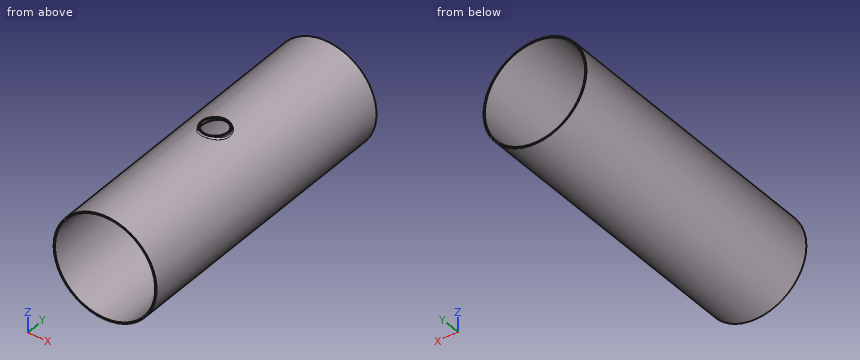
Autodesk Inventor part; units mm, degrees
ref_plane "YZ Plane" through (0, 0, 0) normal (1, 0, 0) x (0, 1, 0)
ref_plane "XZ Plane" through (0, 0, 0) normal (0, 1, 0) x (-1, 0, 0)
ref_plane "XY Plane" through (0, 0, 0) normal (0, 0, 1) x (1, 0, 0)
sketch "Szkic8" plane through (0, 0, 0) normal (0, 1, 0) x (-1, 0, 0)
  circle A0 centre (0, 0) radius 77
  circle A1 centre (0, 0) radius 75
  dimension "d53" = 154
  dimension "d54" = 2
extrude "Wyciągnięcie proste2" add sketch "Szkic8" along normal mid plane 450
sketch "Szkic13" plane through (0, 0, 0) normal (0, 0, 1) x (1, 0, 0)
  circle A0 centre (0, 0) radius 20.5
  circle A1 centre (0, 0) radius 18.5
  dimension "d67" = 41
  dimension "d68" = 2
extrude "Wyciągnięcie proste6" add sketch "Szkic13" along normal blind 79
sketch "Szkic14" plane through (0, 0, 79) normal (0, 0, 1) x (1, 0, 0)
  circle A0 centre (0, 0) radius 18.5
extrude "Wyciągnięcie proste7" cut sketch "Szkic14" against normal blind 79
sketch "Szkic15" plane through (0, -225, 0) normal (0, -1, 0) x (1, 0, 0)
  circle A0 centre (0, 0) radius 75
extrude "Wyciągnięcie proste8" cut sketch "Szkic15" against normal blind 450
fillet "Zaokrąglenie3" radius 2 2 edges at (0, 20.5, 77) (-0.0041, -20.5, 77)
fillet "Zaokrąglenie4" radius 4 2 edges at (-0.0039, -18.5, 75) (0, 18.5, 75)
equation "\"d53\" = OD"
equation "\"d54\" = THK"
equation "\"d55\" = L1"
equation "\"d67\" = OD2"
equation "\"d68\" = THK"
equation "\"d69\" = L2"
equation "\"d71\" = L2"
equation "\"d73\" = L1"
equation "\"d75\" = THK"
equation "\"d76\" = 2 * THK"
equation "\"SzerokośćGięciaPodcięcia\" = Grubość"
equation "\"RozmiarPodcięciaNarożnika\" = 4 * Grubość"
equation "\"PromieńPrzejścia\" = PromieńGięcia"
equation "\"Rozmiar_promienia_Jacobiego\" = PromieńGięcia"
equation "\"Wielk_odstępu\" = Grubość"
equation "\"d2\" = PromieńGięcia"
equation "\"d23\" = PromieńGięcia"
equation "\"OD\" = 154"
equation "\"THK\" = 2"
equation "\"L1\" = 450"
equation "\"L2\" = 79"
equation "\"OD2\" = 41"
properties part number "Trójnik red. krótki  Ø154 41 154 s=2 L=450" material "304"
Part model, mm, in its own coordinate system. Round coordinates to 2 decimals unless told otherwise and drop trailing zeros. Write each loop counter-clockwise with the first axis right and the second up, starting at its lowest first coordinate (ties: lowest second). Pieces come first, ordered by that corner, then holes. Notation, with made-up numbers: M 37.25,-10 L 76.25,-10 A13 cw 76.25,14 Z; hole C 29,71.5 d6. An arc over 180 degrees is marked long. Answer as CSV lines item,"result". Start each with the question number.
1) Band-saw the part on B-B (x = 41). List the corners of the cut face in (y, z), then the cut area to 3 significant figures.
2) Band-saw the part on A-A (z = 0). List the corners of the cut face in (x, y).
3) Drill centre lines: L1, parallel to X at y = 0, z = 77.95; L2, parallel to Z at x = 1, y = -147.5; L3, parallel to Z at x = -34, y = 163.5. Where is each one in solid material? Low to high.
4) Drop flat-ended pins along their axis: pin 1 (6 mm diameter, centred on y = -165.5, z = -12.5, fed in from -X); pin 2 (1.5 mm diameter, centred on x = -18.5, y = 33, fed in from -Z); pin 3 (12 mm diameter, centred on x = -24.5, y = -138, fed in from -Z). Give the stop position or say it passes through.
5) Band-saw the part on C-C (y = 140). List the corners of the cut face in (x, z).
Worked out:
1,outline,"M -225,-65.18 L 225,-65.18 L 225,-62.8 L -225,-62.8 Z; M -225,62.8 L 225,62.8 L 225,65.18 L -225,65.18 Z"
1,area,"2,140 mm²"
2,outline,"M -77,-225 L -75,-225 L -75,225 L -77,225 Z; M 75,-225 L 77,-225 L 77,225 L 75,225 Z"
3,L1,"-20.5 to -18.5, 18.5 to 20.5"
3,L2,"-76.99 to -74.99, 74.99 to 76.99"
3,L3,"-69.09 to -66.85, 66.85 to 69.09"
4,pin 1,"x = -76.41"
4,pin 2,"z = -74.93"
4,pin 3,"z = -74.74"
5,outline,"C 0,0 d154; hole C 0,0 d150"
